Read the model definition and answer for the solid it produces. Units are mm, in the model's axes. Coordinates: 2 decimals unless noted, no trailing zeros. Write each loop counter-clockwise with the first axis right and the second up, starting at its lowest first coordinate (ties: lowest second). Pieces come first, ordered by that corner, then holes. Notation, with made-up numbers: (34.25, 47) -> (93.25, 47) arc R28 ccw to (93.25, 84) -> close; hole circle Ø9 at (54.25, 16). An arc over 180 degrees is marked (long way). Use CSV: the item, a comma, the result in double quotes.
from build123d import *

# Parameters (mm, degrees)
CYLINDER042_R     = 1.8
CYLINDER042_DEPTH = 10
BOX021_W          = 15
BOX021_H          = 8
BOX021_DEPTH      = 5


with BuildPart() as cylinder007:
    # Cylinder042 → Cylinder042 (new body)
    with BuildSketch(Plane(origin=(7.5, 4, 0), x_dir=(1, 0, 0), z_dir=(0, 0, 1))):
        Circle(CYLINDER042_R)
    extrude(amount=CYLINDER042_DEPTH)


with BuildPart() as fusion015:
    # Cone → Cone (revolve)
    with BuildSketch(Plane(origin=(7.5, 4, 2), x_dir=(1, 0, 0), z_dir=(0, -1, 0))):
        Polygon((0, 0), (1.8, 0), (3.3, 3), (0, 3), align=None)
    revolve(axis=Axis((7.5, 4, 2), (0, 0, 1)))

    # Fusion015: union Cylinder007
    add(cylinder007.part)


with BuildPart() as bottom_stop_trigger_cut:
    # Box021 → Box021 (new body)
    with BuildSketch(Plane.XY):
        with Locations((7.5, 4)):
            Rectangle(BOX021_W, BOX021_H)
    extrude(amount=BOX021_DEPTH)

    # Cut015: cut Fusion015
    add(fusion015.part, mode=Mode.SUBTRACT)


solid = bottom_stop_trigger_cut.part
1. A cutting plane is placed at A-A (y = 4). Give the vertices of the cut face in (x, z), and give its area (3 significant figures).
Solutions:
outline,"(0, 0) -> (5.7, 0) -> (5.7, 2) -> (4.2, 5) -> (0, 5) -> close; (9.3, 0) -> (15, 0) -> (15, 5) -> (10.8, 5) -> (9.3, 2) -> close"
area,"52.5 mm^2"
2. For a pull along Y with two mould halves and no side action, classify faces 1 (the cylindrical face through (5.7, 4.08, 0.99)), 2 (the flat face through (15, 4, 2)), 3 (the flat face through (7, 0, 2)) as pulls with the +Y half, pulls with the -Y half, needs draft (parallel to the pull), parting line crosses it, or undercut.
Solutions:
face 1,"undercut"
face 2,"needs draft"
face 3,"pulls with the -Y half"
3. A cutting plane is placed at D-D (z = 1.6). Give the vertices of the cut face in (x, y), and give its area (3 significant figures).
Solutions:
outline,"(0, 0) -> (15, 0) -> (15, 8) -> (0, 8) -> close; hole circle Ø3.6 at (7.5, 4)"
area,"110 mm^2"
4. Each of these flat-tipped pins is pushed along its axis until it touches: pin 1 Ø4.5 at (x, y) = (7.5, 4) entering from +Z; pin 2 Ø1 at (x, z) = (9.5, 2.5) entering from -Y. Where does it stop, or does it pass through?
Solutions:
pin 1,"stops at z = 2.9"
pin 2,"stops at y = 0"
5. Find the intervals of material crossed by line 1 along Y through (x, z) = (7.5, 1.2); line 2 along X through (y, z) = (3.25, 4.45); line 3 along X through (y, z) = (5.5, 2.6), in increasing order.
Solutions:
line 1,"y = 0 to 2.2, 5.8 to 8"
line 2,"x = 0 to 4.57, 10.43 to 15"
line 3,"x = 0 to 6.03, 8.97 to 15"
6. A cutting plane is placed at C-C (z = 3.8). Give the vertices of the cut face in (x, y).
Solutions:
outline,"(0, 0) -> (15, 0) -> (15, 8) -> (0, 8) -> close; hole circle Ø5.4 at (7.5, 4)"
7. A cutting plane is placed at B-B (x = 7.5). Give the vertices of the cut face in (y, z), and give its area (3 significant figures).
Solutions:
outline,"(0, 0) -> (2.2, 0) -> (2.2, 2) -> (0.7, 5) -> (0, 5) -> close; (5.8, 0) -> (8, 0) -> (8, 5) -> (7.3, 5) -> (5.8, 2) -> close"
area,"17.5 mm^2"
